```python
from build123d import *

# Parameters (mm, degrees)
BOSS_EXTRUDE1_DEPTH = 1.25
SKETCH3_R           = 13.25
SKETCH3_R_2         = 10.75
BOSS_EXTRUDE2_DEPTH = 37
SKETCH4_W           = 4
SKETCH4_H           = 65
BOSS_EXTRUDE3_DEPTH = 7.5
SKETCH5_R           = 1.6
CUT_EXTRUDE1_DEPTH  = 7.5
CHAMFER1_SIZE       = 1.5


with BuildPart() as part:
    # Sketch1 → Boss-Extrude1 (new, symmetric)
    with BuildSketch(Plane(origin=(0, 0, 0), x_dir=(1, 0, 0), z_dir=(0, 1, 0))):
        with BuildLine():
            Line((31, 32.5), (31, 29))
            Line((31, 29), (35, 29))
            Line((35, 29), (35, -29))
            Line((35, -29), (31, -29))
            Line((31, -29), (31, -32.5))
            Line((31, -32.5), (-12.51, -32.5))
            ThreePointArc((-12.51, -32.5), (-28.412831509, -25.912831509), (-35, -10.01))
            Line((-35, -10.01), (-35, 10.01))
            ThreePointArc((-35, 10.01), (-28.412831509, 25.912831509), (-12.51, 32.5))
            Line((-12.51, 32.5), (31, 32.5))
        make_face()
    extrude(amount=BOSS_EXTRUDE1_DEPTH, both=True)

    # Sketch3 → Boss-Extrude2 (add)
    with BuildSketch(Plane(origin=(0, 1.25, 0), x_dir=(1, 0, 0), z_dir=(0, 1, 0))):
        with Locations(Location((-12.51, 0, 0), (0, 0, 90))):
            Circle(SKETCH3_R)
        with Locations(Location((-12.51, 0, 0), (0, 0, 270))):
            Circle(SKETCH3_R_2, mode=Mode.SUBTRACT)
    extrude(amount=BOSS_EXTRUDE2_DEPTH)

    # Sketch4 → Boss-Extrude3 (add)
    with BuildSketch(Plane(origin=(0, 1.25, 0), x_dir=(1, 0, 0), z_dir=(0, 1, 0))):
        with Locations((29, 0)):
            Rectangle(SKETCH4_W, SKETCH4_H)
    extrude(amount=BOSS_EXTRUDE3_DEPTH)

    # Sketch5 → Cut-Extrude1 (cut)
    with BuildSketch(Plane.ZY.offset(-27)):
        with Locations((-27.5, 5)):
            Circle(SKETCH5_R)
        with Locations((0, 5)):
            Circle(SKETCH5_R)
        with Locations((27.5, 5)):
            Circle(SKETCH5_R)
    extrude(amount=-CUT_EXTRUDE1_DEPTH, mode=Mode.SUBTRACT)

    # Chamfer1
    chamfer1_edges = [part.edges().sort_by_distance(p)[0] for p in [
        (27, 5, -29.1),
        (27, 5, -1.6),
        (27, 5, 25.9),
    ]]
    chamfer(chamfer1_edges, length=CHAMFER1_SIZE)


solid = part.part
```
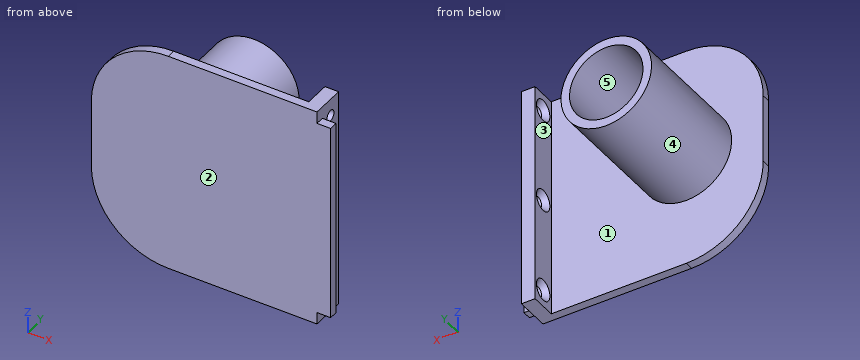
For this review, take the finished solid that the model builds, in its own axes (mm). Face numbers are marked on the shaded views. A direction names the side the tool comes from. Give positions to 0.01 mm unless a question says otherwise; leave off trailing zeros. Order: outer loops, then holes, each group sorted by start corner. A loop starts at its lowest first (then second) coordinate and runs counter-clockwise, first axis right, second up.
1) Take a section at A-A (z = 0). Give the boundary of the cut face in (x, y).
2) The part is to be moulded in two halves that separate along Z. For the marked faces 3, 4 and 5, say which applies: released by +Z, released by -Z, zero draft, split by the parting line, or undercut.
3) Take a section at D-D (y = 21.5). Give the boundary of the cut face in (x, z), then the cut area to 3 significant figures.
4) Wall thickness on line 1 (X direction, y = 10.5, z = 0); line 2 (Y direction, x = 29.75, z = -27.5); line 3 (Y direction, x = 8.5, z = -28.5): over which ranges is each line inside the solid? List them lowest first.
5) For the marked faces 1 and 2, list the 3-axis set-ups (+Z, -Z, +X, -X, +Y, -Y) from which the entire face can be reached by the end or side of a thin tool; tool diameter is ignored.
6) Take a section at B-B (y = 5). Give the boundary of the cut face in (x, z), then the cut area to 3 significant figures.
7) Insertion check: pin 1 (2 mm diameter, centred on x = 34, y = -0.5, fed in from +Z); pin 2 (4.5 mm diameter, centred on x = 33, z = -11, fed in from +Y); pin 3 (5 mm diameter, centred on x = -3, z = -23, fed in from +Y). Each pin has a flat end and moves straight along its axis. Give the tip position at first contact, or say it passes through.
8) Take a section at C-C (x = -8). Give the boundary of the cut face in (y, z).
Derived:
1. outline: (-35, -1.25) - (35, -1.25) - (35, 1.25) - (31, 1.25) - (31, 3.4) - (28.5, 3.4) - (27, 1.9) - (27, 1.25) - (0.74, 1.25) - (0.74, 38.25) - (-1.76, 38.25) - (-1.76, 1.25) - (-23.26, 1.25) - (-23.26, 38.25) - (-25.76, 38.25) - (-25.76, 1.25) - (-35, 1.25) - close; (27, 8.1) - (28.5, 6.6) - (31, 6.6) - (31, 8.75) - (27, 8.75) - close
2. face 3: zero draft
2. face 4: split by the parting line
2. face 5: undercut
3. outline: circle Ø26.5 at (-12.51, 0); hole circle Ø21.5 at (-12.51, 0)
3. area: 188 mm2
4. line 1: x = -25.76 to -23.26, -1.76 to 0.74
4. line 2: y = -1.25 to 3.4, 6.6 to 8.75
4. line 3: y = -1.25 to 1.25
5. face 1: +Y
5. face 2: +Z, -Z, +X, -X, -Y
6. outline: circle Ø26.5 at (-12.51, 0); (27, -32.5) - (31, -32.5) - (31, -29.1) - (28.5, -29.1) - (27, -30.6) - close; (27, -24.4) - (28.5, -25.9) - (31, -25.9) - (31, -1.6) - (28.5, -1.6) - (27, -3.1) - close; (27, 3.1) - (28.5, 1.6) - (31, 1.6) - (31, 25.9) - (28.5, 25.9) - (27, 24.4) - close; (27, 30.6) - (28.5, 29.1) - (31, 29.1) - (31, 32.5) - (27, 32.5) - close; hole circle Ø21.5 at (-12.51, 0)
6. area: 403 mm2
7. pin 1: stops at z = 29
7. pin 2: stops at y = 8.75
7. pin 3: stops at y = 1.25
8. outline: (-1.25, -32.5) - (1.25, -32.5) - (1.25, -12.46) - (38.25, -12.46) - (38.25, -9.76) - (1.25, -9.76) - (1.25, 9.76) - (38.25, 9.76) - (38.25, 12.46) - (1.25, 12.46) - (1.25, 32.5) - (-1.25, 32.5) - close
